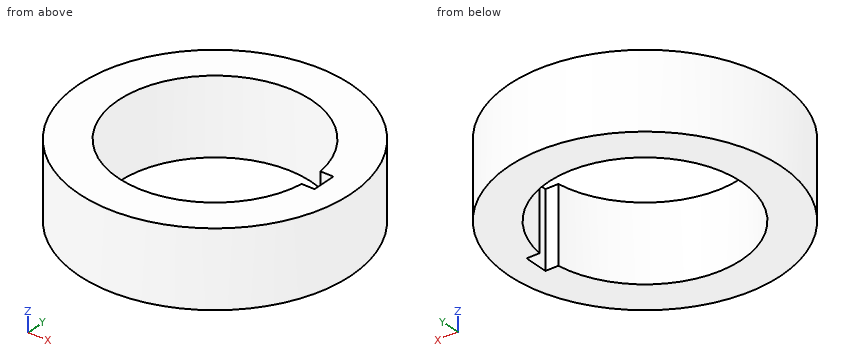
Autodesk Fusion 360 part; units mm, degrees
sketch "Sketch1" plane through (0, 0, 0) normal (0, 0, 1) x (1, 0, 0)
  circle A0 centre (0, 0) radius 16
  line L0 (0, 0) -> (16, 0)
  line L1 (15.8745, -2) -> (18, -2)
  line L2 (18, -2) -> (18, 2)
  line L3 (18, 2) -> (15.8745, 2)
  circle A1 centre (0, 0) radius 22.5
  dimension "d1" = 32
extrude "Extrude1" add sketch "Sketch1" along normal blind 12.5
Verification items for the finished model (mm, model axes). Round coordinates to 2 decimals unless told otherwise and drop trailing zeros. Loops run counter-clockwise (first coordinate to the right, second up) from the corner with the lowest first, then second, coordinate; pieces in that order, holes last. Notation, with made-up numbers: (-5, -26.75) - (16, -26.75) arc R28 ccw to (16, -7.75) - close; hole circle Ø7 at (60.5, 51.25). An arc over 180 degrees is marked (long way). Use a Markdown table: item, result. Add a question column.
1. Section check B-B, the plane y = 0. Record the boundary of the cut face in (x, z).
2. Section check A-A, the plane x = 0. Record the boundary of the cut face in (y, z), plus the area to 4 significant figures.
3. Section check D-D, the plane y = -18.5. Record the boundary of the cut face in (x, z), plus the area to 3 significant figures.
4. Thickness scan on probe 1 along Y at (x, z) = (0, 10.25); probe 2 along X at (y, z) = (0.5, 8); probe 3 along Y at (x, z) = (-7.5, 2.25). Record the ranges inside material, lowest first. Write a range as [from, to].
5. Section check C-C, the plane z = 1.25. Record the boundary of the cut face in (x, y).
6. Gauge pin test, flat ends, axial feed: pin 1 (0.6 mm diameter, centred on x = 17.5, z = 6, fed in from +Y); pin 2 (4 mm diameter, centred on y = -3.5, z = 5, fed in from +X); pin 3 (5 mm diameter, centred on y = -14, z = 9.5, fed in from -X). Record the tip position at first contact, or that the pin passes through.
Checks:
| question | item | result |
|---|---|---|
| 1 | outline | (-22.5, 0) - (-16, 0) - (-16, 12.5) - (-22.5, 12.5) - close; (18, 0) - (22.5, 0) - (22.5, 12.5) - (18, 12.5) - close |
| 2 | outline | (-22.5, 0) - (-16, 0) - (-16, 12.5) - (-22.5, 12.5) - close; (16, 0) - (22.5, 0) - (22.5, 12.5) - (16, 12.5) - close |
| 2 | area | 162.5 mm^2 |
| 3 | outline | (-12.81, 0) - (12.81, 0) - (12.81, 12.5) - (-12.81, 12.5) - close |
| 3 | area | 320 mm^2 |
| 4 | probe 1 | y = [-22.5, -16], [16, 22.5] |
| 4 | probe 2 | x = [-22.49, -15.99], [18, 22.49] |
| 4 | probe 3 | y = [-21.21, -14.13], [14.13, 21.21] |
| 5 | outline | circle Ø45 at (0, 0); hole (15.87, -2) - (18, -2) - (18, 2) - (15.87, 2) arc R16 ccw (long way) to start |
| 6 | pin 1 | stops at y = 14.51 |
| 6 | pin 2 | stops at x = 22.45 |
| 6 | pin 3 | stops at x = -19.34 |
